from build123d import *

# Parameters (mm, degrees)
BOX001_W               = 37
BOX001_H               = 39
BOX001_DEPTH           = 10
BOX001_PLACEMENT_ANGLE = 57
BOX_W                  = 37
BOX_H                  = 39
BOX_DEPTH              = 10
CYLINDER001_R          = 22
CYLINDER001_DEPTH      = 37
CYLINDER_R             = 25
CYLINDER_DEPTH         = 40
CYLINDER004_R          = 21
CYLINDER004_DEPTH      = 21
CYLINDER003_R          = 23
CYLINDER003_DEPTH      = 10
CYLINDER002_R          = 25
CYLINDER002_DEPTH      = 5
FILLET_R               = 4.5


with BuildPart() as cubo001:
    # Box001 → Box001 (new body)
    with BuildSketch(Plane.XY):
        with Locations((18.5, 19.5)):
            Rectangle(BOX001_W, BOX001_H)
    extrude(amount=BOX001_DEPTH)


with BuildPart() as cubo001_1:
    # Box001 placement: moved
    add(cubo001.part.moved(Location((0, 0, 37))).rotate(Axis((0, 0, 37), (0, 0, -1)), BOX001_PLACEMENT_ANGLE))


with BuildPart() as cut002:
    # Box → Box (new body)
    with BuildSketch(Plane.XY.offset(37)):
        with Locations((18.5, 19.5)):
            Rectangle(BOX_W, BOX_H)
    extrude(amount=BOX_DEPTH)

    # Cut002: cut Cubo001
    add(cubo001_1.part, mode=Mode.SUBTRACT)


with BuildPart() as cilindro001:
    # Cylinder001 → Cylinder001 (new body)
    with BuildSketch(Plane.XY):
        Circle(CYLINDER001_R)
    extrude(amount=CYLINDER001_DEPTH)


with BuildPart() as cut:
    # Cylinder → Cylinder (new body)
    with BuildSketch(Plane.XY):
        Circle(CYLINDER_R)
    extrude(amount=CYLINDER_DEPTH)

    # Cut: cut Cilindro001
    add(cilindro001.part, mode=Mode.SUBTRACT)


with BuildPart() as cilindro004:
    # Cylinder004 → Cylinder004 (new body)
    with BuildSketch(Plane.XY):
        Circle(CYLINDER004_R)
    extrude(amount=CYLINDER004_DEPTH)


with BuildPart() as cut001:
    # Cylinder003 → Cylinder003 (new body)
    with BuildSketch(Plane.XY):
        Circle(CYLINDER003_R)
    extrude(amount=CYLINDER003_DEPTH)

    # Cut001: cut Cilindro004
    add(cilindro004.part, mode=Mode.SUBTRACT)


with BuildPart() as cut001_1:
    # Cut001 placement: moved
    add(cut001.part.moved(Location((0, 0, -5))))


with BuildPart() as cut003:
    # Cylinder002 → Cylinder002 (new body)
    with BuildSketch(Plane.XY.offset(40)):
        Circle(CYLINDER002_R)
    extrude(amount=CYLINDER002_DEPTH)

    # Fillet
    fillet_edges = [cut003.edges().sort_by_distance(p)[0] for p in [
        (-25, 0, 45),
    ]]
    fillet(fillet_edges, radius=FILLET_R)

    # Fusion: union Cut, Cut001
    add(cut.part)
    add(cut001_1.part)

    # Cut003: cut Cut002
    add(cut002.part, mode=Mode.SUBTRACT)


solid = cut003.part
The model under review builds one solid part; all positions refer to its coordinate system, in mm. A direction names the side the tool comes from. Round coordinates to 2 decimals unless told otherwise and drop trailing zeros. Write each loop counter-clockwise with the first axis right and the second up, starting at its lowest first coordinate (ties: lowest second). Pieces come first, ordered by that corner, then holes. Notation, with made-up numbers: M -6,87 L 0,87 A5 ccw 0,92 Z; hole C 55.5,-8 d8. An arc over 180 degrees is marked long. Answer as CSV lines item,"result". Start each with the question number.
Q1. Wall thickness on line 1 along X through (y, z) = (0, 13.5); line 2 along X through (y, z) = (0, 2.5): over which ranges is each line inside the solid? List them lowest first.
Q2. Clearance check with flat-ended pins moving along their axes: P1, Ø10.5, axis at x = 15, y = 18.5, coming from the +Z side; P2, Ø1.5, axis at x = -18.5, z = 2.5, coming from the +Y side; P3, Ø3, axis at y = 3, z = 27.5, coming from the -X side; P4, Ø3, axis at x = -1, z = 32.5, coming from the +Y side. State where each tip first meets the part, or that it passes through.
Q3. The part is to be moulded in two halves that separate along X. For faces 3 (the face through (-4.769, -21.477, 20.776)), 4 (the face through (20.03, 6.31, -0.07)), 5 (the face through (-20, -15, 20)), 6 (the face through (-0.3, 0.3, 45)), say which applies: +X half, -X half, draft (parallel to the pull), parting line (faces both ways), or undercut.
Q4. Consider section A-A, the plane z = 28.5. Give the boundary of the cut face in (x, y), then the cut area to 3 significant figures.
Q5. Tool access review of faces 1 (the face through (22.1, -7.3, 0)), 2 (the face through (10, -19, -5)): name each direction out of +Z, -Z, +X, -X, +Y, -Y from which nothing blocks a thin tool from reaching the whole face with its end or side.
Result set:
1,line 1,"x = -25 to -22, 22 to 25"
1,line 2,"x = -25 to -21, 21 to 25"
2,P1,"stops at z = 37"
2,P2,"stops at y = 17.61"
2,P3,"stops at x = -24.95"
2,P4,"stops at y = 25"
3,face 3,"undercut"
3,face 4,"undercut"
3,face 5,"parting line"
3,face 6,"draft"
4,outline,"C 0,0 d50; hole C 0,0 d44"
4,area,"443 mm²"
5,face 1,"-Z"
5,face 2,"-Z, +X, -X, +Y, -Y"
